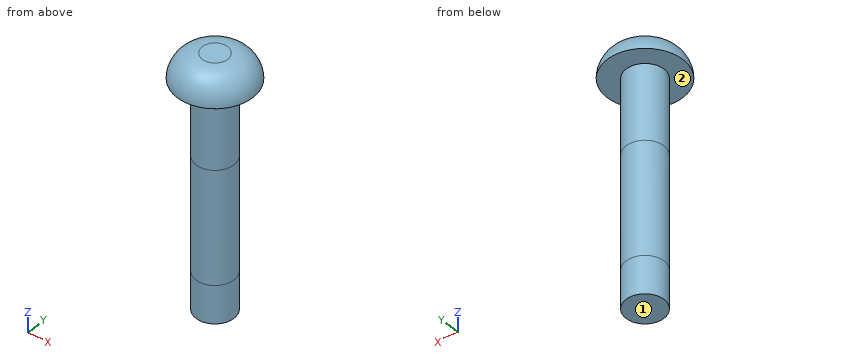
Autodesk Inventor part; units mm, degrees
ref_plane "YZ Plane" through (0, 0, 0) normal (1, 0, 0) x (0, 1, 0)
ref_plane "XZ Plane" through (0, 0, 0) normal (0, 1, 0) x (-1, 0, 0)
ref_plane "XY Plane" through (0, 0, 0) normal (0, 0, 1) x (1, 0, 0)
sketch "スケッチ1" plane through (0, 0, 0) normal (0, 0, 1) x (1, 0, 0)
  circle A0 centre (0, 0) radius 1.5
  dimension "d0" = 3
extrude "押し出し1" add sketch "スケッチ1" along normal blind 6
sketch "スケッチ2" plane through (0, 0, 6) normal (0, 0, 1) x (1, 0, 0)
  circle A0 centre (0, 0) radius 1.5
  circle A1 centre (0, 0) radius 3
  dimension "d3" = 6
extrude "押し出し2" add sketch "スケッチ2" along normal blind 2 contours A0 | A1
fillet "フィレット1" radius 2 1 edges at (-3, 0, 8)
thread "ねじ1"
sketch "スケッチ3" plane through (0, 0, 0) normal (0, 0, -1) x (-1, 0, 0)
  circle A0 centre (0, 0) radius 1.5
extrude "押し出し3" add sketch "スケッチ3" along normal blind 9
sketch "スケッチ4" plane through (0, 0, -9) normal (0, 0, -1) x (-1, 0, 0)
  circle A0 centre (0, 0) radius 1.5
extrude "押し出し4" add sketch "スケッチ4" along normal blind 3
properties part number "SB　18mmなべネジ" material "Steel, Mild"
Build history of the part. All positions in model axes, mm. Face numbers are marked on the shaded views. A direction names the side the tool comes from. Coordinates: 2 decimals unless noted, no trailing zeros. Write each loop counter-clockwise with the first axis right and the second up, starting at its lowest first coordinate (ties: lowest second). Pieces come first, ordered by that corner, then holes.
(1) Drill centre lines: line 1 (Y direction, x = 0, z = 3.5); line 2 (Z direction, x = -1.25, y = 2.25); line 3 (X direction, y = -0.75, z = -9.25). Where is each one in solid material? Low to high.
(2) Pin check, flat tip, straight feed: pin 1 Ø2 at (x, z) = (0.5, -9) entering from -Y. Stop position of the tip, or through.
(3) 3-axis set-ups, long thin cutter, end or side, ignore diameter. For the marked faces 1 and 2: which of +Z, -Z, +X, -X, +Y, -Y reach the whole face in a straight line?
(4) Cut at A-A on z = -8. List the corners of the cut face in (x, y).
Working result:
1. line 1: y = -1.5 to 1.5
1. line 2: z = 6 to 7.23
1. line 3: x = -1.3 to 1.3
2. pin 1: stops at y = -1.5
3. face 1: -Z, +X, -X, +Y, -Y
3. face 2: -Z
4. outline: circle Ø3 at (0, 0)
